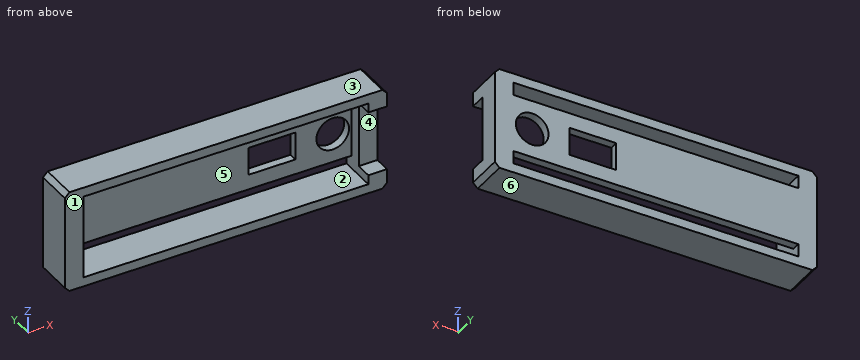
from build123d import *

# Parameters (mm, degrees)
SKETCH1_W                       = 70
SKETCH1_H                       = 12
BOSS_EXTRUDE1_DEPTH             = 1.8
SKETCH2_W                       = 4
SKETCH2_H                       = 18
BOSS_EXTRUDE2_DEPTH             = 8
BOSS_EXTRUDE3_REACH             = 40.58
SKETCH3_W                       = 5
SKETCH3_H                       = 18
BOSS_EXTRUDE3_DIRECTION_2_REACH = 40.58
SKETCH4_W                       = 5
SKETCH4_H                       = 14
CUT_EXTRUDE1_DEPTH              = 3.5
SKETCH5_W                       = 61
SKETCH5_H                       = 12.5
BOSS_EXTRUDE4_DEPTH             = 1.8
SKETCH7_W                       = 70
SKETCH7_H                       = 2
BOSS_EXTRUDE5_DEPTH             = 8
SKETCH10_R                      = 3.5
CUT_EXTRUDE2_DEPTH              = 1.8
SKETCH11_W                      = 10
SKETCH11_H                      = 6
CUT_EXTRUDE3_DEPTH              = 1.8
CUT_EXTRUDE4_START              = -8
SKETCH12_W                      = 1
SKETCH12_H                      = 22
CUT_EXTRUDE4_DEPTH              = 8
CHAMFER1_SIZE                   = 1


with BuildPart() as part:
    # Sketch1 → Boss-Extrude1 (new body)
    with BuildSketch(Plane(origin=(0, 0, 0), x_dir=(1, 0, 0), z_dir=(0, 1, 0))):
        with Locations((0, 6)):
            Rectangle(SKETCH1_W, SKETCH1_H)
    extrude(amount=BOSS_EXTRUDE1_DEPTH)

    # Sketch2 → Boss-Extrude2 (add)
    with BuildSketch(Plane(origin=(0, 1.8, 0), x_dir=(1, 0, 0), z_dir=(0, 1, 0))):
        with Locations((-33, 6)):
            Rectangle(SKETCH2_W, SKETCH2_H)
    extrude(amount=-BOSS_EXTRUDE2_DEPTH)

    # Boss-Extrude3: up to this face of the body (flat: up to its plane)
    boss_extrude3_end = Plane(part.part.faces().sort_by_distance((-33, -6.2, -6))[0])
    # Sketch3 → Boss-Extrude3 (add, up to the picked face)
    with BuildSketch(Plane.XZ, mode=Mode.PRIVATE) as boss_extrude3_sk1:
        with Locations((32.5, -6)):
            Rectangle(SKETCH3_W, SKETCH3_H)
    boss_extrude3_tool1 = split(extrude(boss_extrude3_sk1.sketch, amount=BOSS_EXTRUDE3_REACH, mode=Mode.PRIVATE), bisect_by=boss_extrude3_end, keep=Keep.BOTH, mode=Mode.PRIVATE)
    add(boss_extrude3_tool1.solids().sort_by(Axis((32.5, 0, -6), (0, -1, 0)))[0])

    # Boss-Extrude3 direction 2: up to this face of the body (flat: up to its plane)
    boss_extrude3_direction_2_end = Plane(part.part.faces().sort_by_distance((-0.916666667, 1.8, -6))[0])
    # Sketch3 → Boss-Extrude3 direction 2 (add, up to the picked face)
    with BuildSketch(Plane.XZ, mode=Mode.PRIVATE) as boss_extrude3_direction_2_sk1:
        with Locations((32.5, -6)):
            Rectangle(SKETCH3_W, SKETCH3_H)
    boss_extrude3_direction_2_tool1 = split(extrude(boss_extrude3_direction_2_sk1.sketch, amount=-BOSS_EXTRUDE3_DIRECTION_2_REACH, mode=Mode.PRIVATE), bisect_by=boss_extrude3_direction_2_end, keep=Keep.BOTH, mode=Mode.PRIVATE)
    add(boss_extrude3_direction_2_tool1.solids().sort_by(Axis((32.5, 0, -6), (0, 1, 0)))[0])

    # Sketch4 → Cut-Extrude1 (cut)
    with BuildSketch(Plane.XZ.offset(6.2)):
        with Locations((32.5, -6)):
            Rectangle(SKETCH4_W, SKETCH4_H)
    extrude(amount=-CUT_EXTRUDE1_DEPTH, mode=Mode.SUBTRACT)

    # Sketch5 → Boss-Extrude4 (add)
    with BuildSketch(Plane(origin=(0, 1.8, 0), x_dir=(1, 0, 0), z_dir=(0, 1, 0))):
        with Locations((-0.5, 6)):
            Rectangle(SKETCH5_W, SKETCH5_H)
    extrude(amount=-BOSS_EXTRUDE4_DEPTH)

    # Sketch7 → Boss-Extrude5 (add)
    with BuildSketch(Plane(origin=(0, 1.8, 0), x_dir=(1, 0, 0), z_dir=(0, 1, 0))):
        with Locations((0, 16)):
            Rectangle(SKETCH7_W, SKETCH7_H)
        with Locations((0, -4)):
            Rectangle(SKETCH7_W, SKETCH7_H)
    extrude(amount=-BOSS_EXTRUDE5_DEPTH)

    # Sketch10 → Cut-Extrude2 (cut)
    with BuildSketch(Plane(origin=(0, 1.8, 0), x_dir=(1, 0, 0), z_dir=(0, 1, 0))):
        with Locations(Location((26, 6, 0), (0, 0, 270))):
            Circle(SKETCH10_R)
    extrude(amount=-CUT_EXTRUDE2_DEPTH, mode=Mode.SUBTRACT)

    # Sketch11 → Cut-Extrude3 (cut)
    with BuildSketch(Plane(origin=(0, 1.8, 0), x_dir=(1, 0, 0), z_dir=(0, 1, 0))):
        with Locations((13, 6)):
            Rectangle(SKETCH11_W, SKETCH11_H)
    extrude(amount=-CUT_EXTRUDE3_DEPTH, mode=Mode.SUBTRACT)

    # Sketch12 → Cut-Extrude4 (cut)
    with BuildSketch(Plane(origin=(0, 1.8, 0), x_dir=(1, 0, 0), z_dir=(0, 1, 0)).offset(CUT_EXTRUDE4_START)):
        with Locations((34.5, 6)):
            Rectangle(SKETCH12_W, SKETCH12_H)
    extrude(amount=CUT_EXTRUDE4_DEPTH, mode=Mode.SUBTRACT)

    # Chamfer1
    chamfer1_edges = [part.edges().sort_by_distance(p)[0] for p in [
        (-35, -2.2, -17),
        (-35, -2.2, 5),
        (34, -2.2, 5),
        (34, -2.2, -17),
    ]]
    chamfer(chamfer1_edges, length=CHAMFER1_SIZE)


solid = part.part
The listing builds one solid part. Answer for the finished solid, in the listing's coordinates (mm). Face numbers are marked on the shaded views. A direction names the side the tool comes from. Give positions to 0.01 mm unless a question says otherwise; leave off trailing zeros. Write each loop counter-clockwise with the first axis right and the second up, starting at its lowest first coordinate (ties: lowest second). Pieces come first, ordered by that corner, then holes.
1) Given P1, Ø4, axis at x = 0, z = -8, coming from the -Y side; P2, Ø4, axis at x = 26, z = -6, coming from the -Y side; P3, Ø2, axis at x = 32.5, z = -6, coming from the -Y side, each flat-ended and moving along its own axis, determine where each tip first touches the part or whether it passes through.
2) For a pull along Z with two mould halves and no side action, classify the marked faces 1, 2, 3 and 4 as pulls with the +Z half, pulls with the -Z half, needs draft (parallel to the pull), parting line crosses it, or undercut.
3) Section C-C (z = -13.75) is taken. Write down the section's boundary in (x, y), and give its area (3 significant figures).
4) Section A-A (x = 26) is taken. Write down the section's boundary in (y, z).
5) Find the intervals of material crossed by L1, parallel to X at y = 0.5, z = -6; L2, parallel to Z at x = -9.5, y = 1.5; L3, parallel to Z at x = 20.5, y = -1.5, in increasing order.
6) A tool of negligible diameter and unlimited length cuts with its end or side. For the marked faces 5 and 6, from which of +Z, -Z, +X, -X, +Y, -Y can it reach the whole face along a straight path? Write none if from no direction.
7) Section B-B (z = -6) is taken. Write down the section's boundary in (x, y).
8) Section D-D (y = -4) is taken. Write down the section's boundary in (x, z), and give its area (3 significant figures).
Response:
1. P1: stops at y = 0
1. P2: passes through
1. P3: stops at y = -2.7
2. face 1: needs draft
2. face 2: undercut
2. face 3: pulls with the +Z half
2. face 4: undercut
3. outline: (-35, -6.2) - (-31, -6.2) - (-31, 1.8) - (-35, 1.8) - close; (30, -6.2) - (34, -6.2) - (34, 1.8) - (30, 1.8) - close
3. area: 64.0 mm2
4. outline: (-6.2, -17) - (1.8, -17) - (1.8, -15) - (-6.2, -15) - close; (-6.2, 3) - (1.8, 3) - (1.8, 5) - (-6.2, 5) - close; (0, -12.25) - (1.8, -12.25) - (1.8, -9.5) - (0, -9.5) - close; (0, -2.5) - (1.8, -2.5) - (1.8, 0.25) - (0, 0.25) - close
5. L1: x = -35 to 8, 18 to 22.5, 29.5 to 34
5. L2: z = -17 to -15, -12.25 to 0.25, 3 to 5
5. L3: z = -17 to -15, 3 to 5
6. face 5: -Y
6. face 6: -Z, +X, -X, +Y, -Y
7. outline: (-35, -6.2) - (-31, -6.2) - (-31, 0) - (8, 0) - (8, 1.8) - (-35, 1.8) - close; (18, 0) - (22.5, 0) - (22.5, 1.8) - (18, 1.8) - close; (29.5, 0) - (30, 0) - (30, -2.7) - (34, -2.7) - (34, 1.8) - (29.5, 1.8) - close
8. outline: (-35, -16) - (-34, -17) - (33, -17) - (34, -16) - (34, -13) - (30, -13) - (30, -15) - (-31, -15) - (-31, 3) - (30, 3) - (30, 1) - (34, 1) - (34, 4) - (33, 5) - (-34, 5) - (-35, 4) - close
8. area: 362 mm2
